Read the model definition and answer for the solid it produces. Units are mm, in the model's axes. A direction names the side the tool comes from. Round coordinates to 2 decimals unless told otherwise and drop trailing zeros. Loops run counter-clockwise (first coordinate to the right, second up) from the corner with the lowest first, then second, coordinate; pieces in that order, holes last. Notation, with made-up numbers: (2, -15) -> (15, -15) arc R25 cw to (15, 9) -> close; hole circle Ø10 at (34, 85). An arc over 180 degrees is marked (long way). Put each result on its own line as item: value.
from build123d import *

# Parameters (mm, degrees)
SKETCH1_R           = 1.175004
SKETCH1_R_2         = 2.4892
SKETCH1_R_3         = 3.175
SKETCH1_W           = 63.5
SKETCH1_H           = 63.5
BOSS_EXTRUDE1_DEPTH = 6.35
SKETCH3_R           = 3.175
CUT_EXTRUDE1_DEPTH  = 6.35


with BuildPart() as part:
    # Sketch1 → Boss-Extrude1 (new body)
    with BuildSketch(Plane(origin=(0, 0, 0), x_dir=(1, 0, 0), z_dir=(0, 1, 0))):
        Polygon((-107.95, -73.66), (107.95, -73.66), (107.95, -26.9875), (40.462499974, -26.9875), (35.699999974, -26.924), (35.699999974, 26.924), (40.462499974, 26.9875), (107.95, 26.9875), (107.95, 73.66), (-107.95, 73.66), (-125.73, 73.66), (-125.73, -73.66), align=None)
        with Locations(Location((0.750006374, -31.75, 0), (0, 0, 270))):
            Circle(SKETCH1_R, mode=Mode.SUBTRACT)
        with Locations(Location((26.174999974, 6.35, 0), (0, 0, 270))):
            Circle(SKETCH1_R_2, mode=Mode.SUBTRACT)
        with Locations(Location((26.174999974, -6.35, 0), (0, 0, 90))):
            Circle(SKETCH1_R_2, mode=Mode.SUBTRACT)
        with Locations(Location((-8.750000026, -31.75, 0), (0, 0, 270))):
            Circle(SKETCH1_R, mode=Mode.SUBTRACT)
        with Locations(Location((-94.475000026, -41.275, 0), (0, 0, 90))):
            Circle(SKETCH1_R_3, mode=Mode.SUBTRACT)
        with Locations(Location((-24.625000026, -41.275, 0), (0, 0, 90))):
            Circle(SKETCH1_R_3, mode=Mode.SUBTRACT)
        with Locations(Location((-8.750000026, 31.75, 0), (0, 0, 90))):
            Circle(SKETCH1_R, mode=Mode.SUBTRACT)
        with Locations(Location((-94.475000026, 41.275, 0), (0, 0, 270))):
            Circle(SKETCH1_R_3, mode=Mode.SUBTRACT)
        with Locations(Location((-24.625000026, 41.275, 0), (0, 0, 270))):
            Circle(SKETCH1_R_3, mode=Mode.SUBTRACT)
        with Locations(Location((0.750006374, 31.75, 0), (0, 0, 90))):
            Circle(SKETCH1_R, mode=Mode.SUBTRACT)
        with BuildLine():
            Line((79.502, 37.592), (92.202, 37.592))
            ThreePointArc((92.202, 37.592), (95.377, 40.767), (92.202, 43.942))
            Line((92.202, 43.942), (79.502, 43.942))
            ThreePointArc((79.502, 43.942), (76.327, 40.767), (79.502, 37.592))
        make_face(mode=Mode.SUBTRACT)
        with BuildLine():
            Line((41.402, 37.592), (54.102, 37.592))
            ThreePointArc((54.102, 37.592), (57.277, 40.767), (54.102, 43.942))
            Line((54.102, 43.942), (41.402, 43.942))
            ThreePointArc((41.402, 43.942), (38.227, 40.767), (41.402, 37.592))
        make_face(mode=Mode.SUBTRACT)
        with BuildLine():
            Line((79.502, -43.942), (92.202, -43.942))
            ThreePointArc((92.202, -43.942), (95.377, -40.767), (92.202, -37.592))
            Line((92.202, -37.592), (79.502, -37.592))
            ThreePointArc((79.502, -37.592), (76.327, -40.767), (79.502, -43.942))
        make_face(mode=Mode.SUBTRACT)
        with BuildLine():
            Line((41.402, -37.592), (54.102, -37.592))
            ThreePointArc((54.102, -37.592), (57.277, -40.767), (54.102, -43.942))
            Line((54.102, -43.942), (41.402, -43.942))
            ThreePointArc((41.402, -43.942), (38.227, -40.767), (41.402, -37.592))
        make_face(mode=Mode.SUBTRACT)
        with Locations((-59.550000026, 0)):
            Rectangle(SKETCH1_W, SKETCH1_H, mode=Mode.SUBTRACT)
    extrude(amount=BOSS_EXTRUDE1_DEPTH)

    # Sketch3 → Cut-Extrude1 (cut)
    with BuildSketch(Plane(origin=(0, 6.35, 0), x_dir=(1, 0, 0), z_dir=(0, 1, 0))):
        with Locations(Location((-115.57, 29.21, 0), (0, 0, 270))):
            Circle(SKETCH3_R)
        with Locations(Location((-115.57, -29.21, 0), (0, 0, 270))):
            Circle(SKETCH3_R)
        with Locations(Location((68.58, 63.5, 0), (0, 0, 270))):
            Circle(SKETCH3_R)
        with Locations(Location((68.58, -63.5, 0), (0, 0, 270))):
            Circle(SKETCH3_R)
    extrude(amount=-CUT_EXTRUDE1_DEPTH, mode=Mode.SUBTRACT)


solid = part.part
Item 1: Which of the six approach directions +Z, -Z, +X, -X, +Y, -Y give full straight-line access (tool end or side, diameter ignored) to faces 1 (the flat face through (-11, 6.35, -1)), 2 (the cylindrical face through (95.376, 3.131, -40.697)), 3 (the flat face through (35.7, 3, 0))?
Derived:
face 1: +Z, -Z, +X, -X, +Y
face 2: +Y, -Y
face 3: +X, +Y, -Y
Item 2: The part is cut by section A-A (z = 63.5). Determine the outline of the cut face in (x, y) (3 decimals).
Derived:
outline: (-125.73, 0) -> (65.405, 0) -> (65.405, 6.35) -> (-125.73, 6.35) -> close; (71.755, 0) -> (107.95, 0) -> (107.95, 6.35) -> (71.755, 6.35) -> close
Item 3: The part is cut by section C-C (z = 6.35). Determine the outline of the cut face in (x, y), then the cut area to 3 significant figures.
Derived:
outline: (-125.73, 0) -> (-91.3, 0) -> (-91.3, 6.35) -> (-125.73, 6.35) -> close; (-27.8, 0) -> (23.69, 0) -> (23.69, 6.35) -> (-27.8, 6.35) -> close; (28.66, 0) -> (35.7, 0) -> (35.7, 6.35) -> (28.66, 6.35) -> close
area: 590 mm^2
Item 4: The part is cut by section B-B (x = 68.58). State how many separate pieces and enclosed holes the cut face has, then the cut area to 3 significant figures.
Derived:
separate pieces: 4
enclosed holes: 0
area: 512 mm^2
Item 5: Find the intervals of material crossed by line 1 along X through (y, z) = (5.25, 6); line 2 along X through (y, z) = (4.5, 15); line 3 along Z through (x, y) = (-8.75, 1.5) (3 decimals), in increasing order.
Derived:
line 1: x = -125.73 to -91.3, -27.8 to 23.71, 28.64 to 35.7
line 2: x = -125.73 to -91.3, -27.8 to 35.7
line 3: z = -73.66 to -32.925, -30.575 to 30.575, 32.925 to 73.66
Item 6: For a pull along X with two mould halves and no side action, classify faces 4 (the flat face through (107.95, 3, -50)), 5 (the flat face through (-11, 0, -1)), 6 (the cylindrical face through (57.276, 3.131, 40.697)) as pulls with the +X half, pulls with the -X half, needs draft (parallel to the pull), parting line crosses it, or undercut.
Derived:
face 4: pulls with the +X half
face 5: needs draft
face 6: undercut
Item 7: The part is cut by section D-D (x = -79). Determine the outline of the cut face in (y, z), then the cut area to 3 significant figures.
Derived:
outline: (0, -73.66) -> (6.35, -73.66) -> (6.35, -31.75) -> (0, -31.75) -> close; (0, 31.75) -> (6.35, 31.75) -> (6.35, 73.66) -> (0, 73.66) -> close
area: 532 mm^2
